Source: CAD feature listing. Evaluate the final solid. Frame: model axes, mm. A direction names the side the tool comes from. Give positions to 0.01 mm unless a question says otherwise; leave off trailing zeros. Order: outer loops, then holes, each group sorted by start corner. A loop starts at its lowest first (then second) coordinate and runs counter-clockwise, first axis right, second up.
1) First-contact query: P1, Ø8, axis at y = -12.5, z = 34.5, coming from the -X side; P2, Ø4, axis at y = 7, z = 9, coming from the +X side; P3, Ø2, axis at y = 9, z = 9, coming from the +X side; P4, Ø6, axis at x = -66.5, y = 15.5, coming from the -Z side. Flat tips, straight axial feed; report the tip coordinate or a pass-through.
2) Section C-C, the plane x = 90.5. Return loops of the section in (y, z), plus the area to 3 significant figures.
3) Draft query along Y for faces 4 (the face through (44.45, 0, 46)), 5 (the face through (-115.44, 1, 12.52)), 6 (the face through (-102.544, 5.199, 12.522)), 7 (the face through (-1, -38.669, 13)). Return one class per face: released by +Y, released by -Y, zero draft, split by the parting line, or undercut.
4) Section B-B, the plane x = 31. Return loops of the section in (y, z).
5) Section A-A, the plane y = 0. Return loops of the section in (x, z).
6) Access query for faces 1 (the face through (26.994, -4.432, 50.519)), 2 (the face through (-44.45, 0, 46)), 3 (the face through (-10.033, 0, 61)). Directions: +Z, -Z, +X, -X, +Y, -Y. A direction counts if a zero-diameter tool reaches every point of the face in a straight line with its end or side. Return the directions, or none.
7) Section D-D, the plane x = 3.5. Return loops of the section in (y, z).
8) Material intervals for line 1 (Z direction, x = 25.5, y = 0); line 2 (X direction, y = -5.5, z = 4); line 3 (Z direction, x = 23.5, y = -23), sorted ascending.
```python
from build123d import *

# Parameters (mm, degrees)
F1_DEPTH      = 25.4
F2_R          = 12.7177056433
F2_R_2        = 12.1311661923
F3_DEPTH      = 25.401
F5_DEPTH      = 44.45
F5_DEPTH_BACK = 44.45
F7_DEPTH      = 25.4
F7_DEPTH_BACK = 25.4
F8_R          = 5.5849461746
F9_DEPTH      = 115.4465217498
F9_DEPTH_BACK = 68.58


with BuildPart() as f1:
    # F0 (on Top) → F1 (new body)
    with BuildSketch(Plane.XY):
        with BuildLine():
            Line((76.2133896351, 39.2316170037), (-76.4946267009, 39.2316170037))
            ThreePointArc((-76.4946267009, 39.2316170037), (-115.4452679188, 0.1401025055), (-76.2133896351, -38.6691577733))
            Line((-76.2133896351, -38.6691577733), (76.2133896351, -38.6691577733))
            ThreePointArc((76.2133896351, -38.6691577733), (115.1637770236, 0.2812296152), (76.2133896351, 39.2316170037))
        make_face()
    extrude(amount=F1_DEPTH)

    # F2 (on Top) → F3 (cut, through all)
    with BuildSketch(Plane.XY):
        with Locations((-89.8385569453, 4.6402988955)):
            Circle(F2_R)
        with Locations((85.2755606174, 4.6516866423)):
            Circle(F2_R_2)
    extrude(amount=F3_DEPTH, mode=Mode.SUBTRACT)

    # F4 (on Right) → F5 (join, two sides)
    with BuildSketch(Plane.YZ) as f5_sk:
        with BuildLine():
            Line((10.6150543281, 54.8590188052), (10.6243238001, 55.3027279675))
            ThreePointArc((10.6243238001, 55.3027279675), (-0.0164444689, 65.9270390411), (-10.6242728941, 55.2698390691))
            ThreePointArc((-10.6242728941, 55.2698390691), (-0.2054618402, 44.6803910476), (10.6150543281, 54.8590188052))
        make_face()
        with BuildLine():
            ThreePointArc((10.6150543281, 54.8590188052), (10.6220061793, 55.0808249798), (10.6243238001, 55.3027279675))
            Line((10.6243238001, 55.3027279675), (10.6150543281, 54.8590188052))
        make_face()
        with BuildLine():
            ThreePointArc((10.6150543281, 54.8590188052), (-0.2054618402, 44.6803910476), (-10.6242728941, 55.2698390691))
            Line((-10.6242728941, 55.2698390691), (-10.4871375507, 10.9702917508))
            Line((-10.4871375507, 10.9702917508), (9.6981804819, 10.9702917508))
            Line((9.6981804819, 10.9702917508), (10.6150543281, 54.8590188052))
        make_face()
    extrude(amount=F5_DEPTH)
    extrude(f5_sk.sketch, amount=-F5_DEPTH_BACK)

    # F6 (on Front) → F7 (cut, two sides)
    with BuildSketch(Plane.XZ) as f7_sk:
        with BuildLine():
            Line((-10.0329583581, 46.5069847835), (-10.0329583581, 44.7021064626))
            ThreePointArc((-10.0329583581, 44.7021064626), (-0.3878303842, 35.5385515118), (9.9337786678, 43.9328126198))
            Line((9.9337786678, 43.9328126198), (9.9920310872, 46.8828118731))
            ThreePointArc((9.9920310872, 46.8828118731), (-0.1890244976, 55.676234637), (-10.0329583581, 46.5069847835))
        make_face()
        with BuildLine():
            ThreePointArc((-10.0329583581, 46.5069847835), (-10.0734626546, 45.6045456231), (-10.0329583581, 44.7021064626))
            Line((-10.0329583581, 44.7021064626), (-10.0329583581, 46.5069847835))
        make_face()
        with BuildLine():
            Line((9.9920310872, 46.8828118731), (9.9337786678, 43.9328126198))
            ThreePointArc((9.9337786678, 43.9328126198), (10.038480918, 44.7657663239), (10.0734626546, 45.6045456231))
            ThreePointArc((10.0734626546, 45.6045456231), (10.0530841501, 46.2449743283), (9.9920310872, 46.8828118731))
        make_face()
        with BuildLine():
            Line((-10.0329583581, 72.3900050139), (-10.0329583581, 46.5069847835))
            ThreePointArc((-10.0329583581, 46.5069847835), (-0.1890244976, 55.676234637), (9.9920310872, 46.8828118731))
            Line((9.9920310872, 46.8828118731), (10.495711118, 72.3900050139))
            Line((10.495711118, 72.3900050139), (-10.0329583581, 72.3900050139))
        make_face()
    extrude(amount=-F7_DEPTH, mode=Mode.SUBTRACT)
    extrude(f7_sk.sketch, amount=F7_DEPTH_BACK, mode=Mode.SUBTRACT)

    # F8 (on Right) → F9 (cut, two sides)
    with BuildSketch(Plane.YZ) as f9_sk:
        with Locations((0, 53.9172701538)):
            Circle(F8_R)
    extrude(amount=-F9_DEPTH, mode=Mode.SUBTRACT)
    extrude(f9_sk.sketch, amount=F9_DEPTH_BACK, mode=Mode.SUBTRACT)


solid = f1.part
```
From the geometry:
1. P1: stops at x = -44.45
1. P2: stops at x = 114.88
1. P3: stops at x = 114.39
1. P4: stops at z = 0
2. outline: (-35.95, 0) - (-6.3, 0) - (-6.3, 25.4) - (-35.95, 25.4) - close; (15.6, 0) - (36.52, 0) - (36.52, 25.4) - (15.6, 25.4) - close
2. area: 1,280 mm2
3. face 4: zero draft
3. face 5: split by the parting line
3. face 6: undercut
3. face 7: released by -Y
4. outline: (-38.67, 0) - (39.23, 0) - (39.23, 25.4) - (10, 25.4) - (10.62, 54.86) arc R10.62 ccw (long way) to (-10.62, 55.27) - (-10.53, 25.4) - (-38.67, 25.4) - close; hole circle Ø11.17 at (0, 53.92)
5. outline: (-115.44, 0) - (-101.68, 0) - (-101.68, 25.4) - (-115.44, 25.4) - close; (-78, 0) - (74.07, 0) - (74.07, 25.4) - (44.45, 25.4) - (44.45, 48.33) - (10.02, 48.33) - (9.99, 46.88) arc R10.07 cw (long way) to (-10.03, 46.51) - (-10.03, 48.33) - (-44.45, 48.33) - (-44.45, 25.4) - (-78, 25.4) - close; (-44.45, 59.5) - (-10.03, 59.5) - (-10.03, 65.93) - (-44.45, 65.93) - close; (10.24, 59.5) - (44.45, 59.5) - (44.45, 65.93) - (10.37, 65.93) - close; (96.48, 0) - (115.16, 0) - (115.16, 25.4) - (96.48, 25.4) - close
6. face 1: +X, -X
6. face 2: +Z, -X, +Y, -Y
6. face 3: +Z, +Y, -Y
7. outline: (-38.67, 0) - (39.23, 0) - (39.23, 25.4) - (10, 25.4) - (10.22, 36.16) - (-10.57, 36.16) - (-10.53, 25.4) - (-38.67, 25.4) - close
8. line 1: z = 0 to 48.33, 59.5 to 65.93
8. line 2: x = -115.01 to -97.51, -82.16 to 78.63, 91.92 to 114.73
8. line 3: z = 0 to 25.4
